Check sheet for the drawn part. Datum: minimum x, y, z corner. Units: mm. A direction names the side the tool comes from. Coordinates: 2 decimals unless noted, no trailing zeros. Order: outer loops, then holes, each group sorted by start corner. A loop starts at its lowest first (then second) coordinate and runs counter-clockwise, first axis right, second up.
Q1. Cross-section at A-A, the plane z = 8.75. Record the boundary of the cut face in (x, y), and give its area (3 significant figures).
Q2. Cross-section at B-B, the plane y = 11. Record the boundary of the cut face in (x, z).
Q3. Draft check along Y on the marked faces 4, 5 and 6. Enter one of: pulls with the +Y half, pulls with the -Y half, needs draft (parallel to the pull), parting line crosses it, or undercut.
Q4. Set-up check for the marked faces 1, 2 and 3: record each of +Z, -Z, +X, -X, +Y, -Y from which the full face is reachable in a straight line by a thin tool's end or side.
Q5. Cross-section at C-C, the plane z = 16. Record the boundary of the cut face in (x, y) (1 decimal).
Q6. Depth check by flat-ended pin: P1, Ø3, axis at x = 4, z = 8.5, coming from the +Y side; P2, Ø11, axis at x = 11, y = 25, coming from the -Z side; P3, Ø5, axis at x = 5.5, z = 11.5, coming from the +Y side; P4, Ø4, axis at x = 12, z = 14, coming from the +Y side. Enter the tip coordinate at first touch or a pass-through.
Q7. Thickness scan on line 1 (Y direction, x = 4.2, z = 4); line 2 (X direction, y = 3, z = 10.75); line 3 (Y direction, x = 11, z = 16.75). Record the ranges inside material, lowest first.
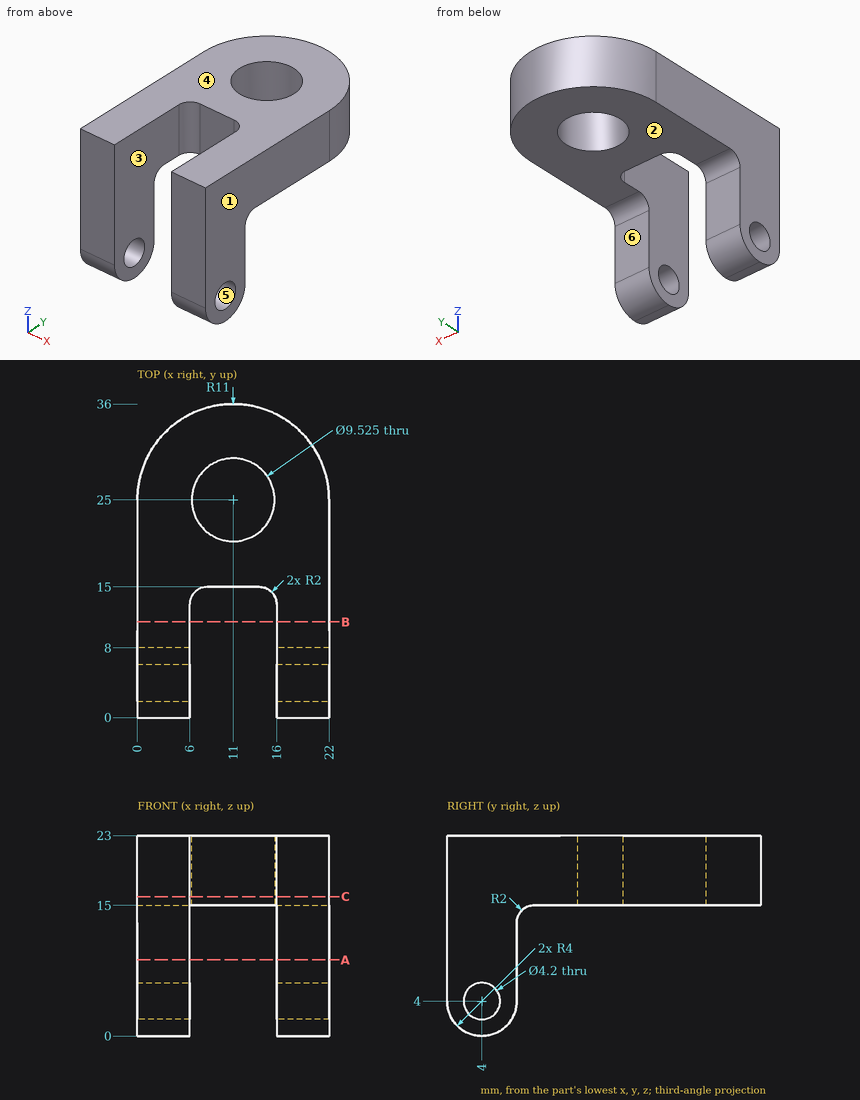
Check values:
1. outline: (0, 0) - (6, 0) - (6, 8) - (0, 8) - close; (16, 0) - (22, 0) - (22, 8) - (16, 8) - close
1. area: 96.0 mm2
2. outline: (0, 15) - (6, 15) - (6, 23) - (0, 23) - close; (16, 15) - (22, 15) - (22, 23) - (16, 23) - close
3. face 4: needs draft
3. face 5: undercut
3. face 6: pulls with the +Y half
4. face 1: +Z, -Z, +X, +Y, -Y
4. face 2: -Z, +X, -X, +Y
4. face 3: +Z, -Z, -Y
5. outline: (0, 0) - (6, 0) - (6, 13) arc R2 cw to (8, 15) - (14, 15) arc R2 cw to (16, 13) - (16, 0) - (22, 0) - (22, 25) arc R11 ccw to (0, 25) - close; hole circle Ø9.5 at (11, 25)
6. P1: stops at y = 8
6. P2: stops at z = 15
6. P3: stops at y = 8.27
6. P4: stops at y = 36
7. line 1: y = 0 to 1.9, 6.1 to 8
7. line 2: x = 0 to 6, 16 to 22
7. line 3: y = 15 to 20.24, 29.76 to 36
